```python
from build123d import *

# Parameters (mm, degrees)
F0_R     = 166
F0_R_2   = 140
F1_DEPTH = 49
F2_DEPTH = 49
F3_DEPTH = 22
F4_DEPTH = 43


with BuildPart() as f1:
    # F0 (on Top) → F1 (new body)
    with BuildSketch(Plane.XY):
        Circle(F0_R)
        Circle(F0_R_2, mode=Mode.SUBTRACT)
    extrude(amount=F1_DEPTH)

    # F0 (on Top) → F2 (join)
    with BuildSketch(Plane.XY):
        Circle(F0_R)
        Circle(F0_R_2, mode=Mode.SUBTRACT)
    extrude(amount=-F2_DEPTH)

    # F0 (on Top) → F3 (join)
    with BuildSketch(Plane.XY):
        with BuildLine():
            ThreePointArc((166.7243233605, -38), (169.9277188905, -19.1198941598), (171, 0))
            ThreePointArc((171, 0), (169.9277188905, 19.1198941598), (166.7243233605, 38))
            ThreePointArc((166.7243233605, 38), (120.9152595829, 120.9152595829), (38, 166.7243233605))
            ThreePointArc((38, 166.7243233605), (19.1198941598, 169.9277188905), (0, 171))
            ThreePointArc((0, 171), (-19.1198941598, 169.9277188905), (-38, 166.7243233605))
            ThreePointArc((-38, 166.7243233605), (-120.9152595829, 120.9152595829), (-166.7243233605, 38))
            ThreePointArc((-166.7243233605, 38), (-169.9277188905, 19.1198941598), (-171, 0))
            ThreePointArc((-171, 0), (-169.9277188905, -19.1198941598), (-166.7243233605, -38))
            ThreePointArc((-166.7243233605, -38), (-120.9152595829, -120.9152595829), (-38, -166.7243233605))
            ThreePointArc((-38, -166.7243233605), (-19.1198941598, -169.9277188905), (0, -171))
            ThreePointArc((0, -171), (19.1198941598, -169.9277188905), (38, -166.7243233605))
            ThreePointArc((38, -166.7243233605), (120.9152595829, -120.9152595829), (166.7243233605, -38))
        make_face()
        Circle(F0_R, mode=Mode.SUBTRACT)
        with BuildLine():
            Line((-316, -38), (-166.7243233605, -38))
            ThreePointArc((-166.7243233605, -38), (-169.9277188905, -19.1198941598), (-171, 0))
            Line((-171, 0), (-326, 0))
            ThreePointArc((-326, 0), (-323.4581542767, -19.6468827044), (-316, -38))
        make_face()
        with BuildLine():
            ThreePointArc((-171, 0), (-169.9277188905, 19.1198941598), (-166.7243233605, 38))
            Line((-166.7243233605, 38), (-316, 38))
            ThreePointArc((-316, 38), (-323.4581542767, 19.6468827044), (-326, 0))
            Line((-326, 0), (-171, 0))
        make_face()
        with BuildLine():
            ThreePointArc((-38, 166.7243233605), (-19.1198941598, 169.9277188905), (0, 171))
            Line((0, 171), (0, 326))
            ThreePointArc((0, 326), (-19.6468827044, 323.4581542767), (-38, 316))
            Line((-38, 316), (-38, 166.7243233605))
        make_face()
        with BuildLine():
            ThreePointArc((0, 171), (19.1198941598, 169.9277188905), (38, 166.7243233605))
            Line((38, 166.7243233605), (38, 316))
            ThreePointArc((38, 316), (19.6468827044, 323.4581542767), (0, 326))
            Line((0, 326), (0, 171))
        make_face()
        with BuildLine():
            ThreePointArc((166.7243233605, 38), (169.9277188905, 19.1198941598), (171, 0))
            Line((171, 0), (326, 0))
            ThreePointArc((326, 0), (323.4581542767, 19.6468827044), (316, 38))
            Line((316, 38), (166.7243233605, 38))
        make_face()
        with BuildLine():
            Line((326, 0), (171, 0))
            ThreePointArc((171, 0), (169.9277188905, -19.1198941598), (166.7243233605, -38))
            Line((166.7243233605, -38), (316, -38))
            ThreePointArc((316, -38), (323.4581542767, -19.6468827044), (326, 0))
        make_face()
        with BuildLine():
            Line((38, -316), (38, -166.7243233605))
            ThreePointArc((38, -166.7243233605), (19.1198941598, -169.9277188905), (0, -171))
            Line((0, -171), (0, -326))
            ThreePointArc((0, -326), (19.6468827044, -323.4581542767), (38, -316))
        make_face()
        with BuildLine():
            Line((0, -326), (0, -171))
            ThreePointArc((0, -171), (-19.1198941598, -169.9277188905), (-38, -166.7243233605))
            Line((-38, -166.7243233605), (-38, -316))
            ThreePointArc((-38, -316), (-19.6468827044, -323.4581542767), (0, -326))
        make_face()
    extrude(amount=F3_DEPTH)

    # F0 (on Top) → F4 (join)
    with BuildSketch(Plane.XY):
        with BuildLine():
            ThreePointArc((-171, 0), (-169.9277188905, 19.1198941598), (-166.7243233605, 38))
            Line((-166.7243233605, 38), (-316, 38))
            ThreePointArc((-316, 38), (-323.4581542767, 19.6468827044), (-326, 0))
            Line((-326, 0), (-171, 0))
        make_face()
        with BuildLine():
            Line((-316, -38), (-166.7243233605, -38))
            ThreePointArc((-166.7243233605, -38), (-169.9277188905, -19.1198941598), (-171, 0))
            Line((-171, 0), (-326, 0))
            ThreePointArc((-326, 0), (-323.4581542767, -19.6468827044), (-316, -38))
        make_face()
        with BuildLine():
            ThreePointArc((166.7243233605, -38), (169.9277188905, -19.1198941598), (171, 0))
            ThreePointArc((171, 0), (169.9277188905, 19.1198941598), (166.7243233605, 38))
            ThreePointArc((166.7243233605, 38), (120.9152595829, 120.9152595829), (38, 166.7243233605))
            ThreePointArc((38, 166.7243233605), (19.1198941598, 169.9277188905), (0, 171))
            ThreePointArc((0, 171), (-19.1198941598, 169.9277188905), (-38, 166.7243233605))
            ThreePointArc((-38, 166.7243233605), (-120.9152595829, 120.9152595829), (-166.7243233605, 38))
            ThreePointArc((-166.7243233605, 38), (-169.9277188905, 19.1198941598), (-171, 0))
            ThreePointArc((-171, 0), (-169.9277188905, -19.1198941598), (-166.7243233605, -38))
            ThreePointArc((-166.7243233605, -38), (-120.9152595829, -120.9152595829), (-38, -166.7243233605))
            ThreePointArc((-38, -166.7243233605), (-19.1198941598, -169.9277188905), (0, -171))
            ThreePointArc((0, -171), (19.1198941598, -169.9277188905), (38, -166.7243233605))
            ThreePointArc((38, -166.7243233605), (120.9152595829, -120.9152595829), (166.7243233605, -38))
        make_face()
        Circle(F0_R, mode=Mode.SUBTRACT)
        with BuildLine():
            Line((0, -326), (0, -171))
            ThreePointArc((0, -171), (-19.1198941598, -169.9277188905), (-38, -166.7243233605))
            Line((-38, -166.7243233605), (-38, -316))
            ThreePointArc((-38, -316), (-19.6468827044, -323.4581542767), (0, -326))
        make_face()
        with BuildLine():
            Line((38, -316), (38, -166.7243233605))
            ThreePointArc((38, -166.7243233605), (19.1198941598, -169.9277188905), (0, -171))
            Line((0, -171), (0, -326))
            ThreePointArc((0, -326), (19.6468827044, -323.4581542767), (38, -316))
        make_face()
        with BuildLine():
            Line((326, 0), (171, 0))
            ThreePointArc((171, 0), (169.9277188905, -19.1198941598), (166.7243233605, -38))
            Line((166.7243233605, -38), (316, -38))
            ThreePointArc((316, -38), (323.4581542767, -19.6468827044), (326, 0))
        make_face()
        with BuildLine():
            ThreePointArc((166.7243233605, 38), (169.9277188905, 19.1198941598), (171, 0))
            Line((171, 0), (326, 0))
            ThreePointArc((326, 0), (323.4581542767, 19.6468827044), (316, 38))
            Line((316, 38), (166.7243233605, 38))
        make_face()
        with BuildLine():
            ThreePointArc((0, 171), (19.1198941598, 169.9277188905), (38, 166.7243233605))
            Line((38, 166.7243233605), (38, 316))
            ThreePointArc((38, 316), (19.6468827044, 323.4581542767), (0, 326))
            Line((0, 326), (0, 171))
        make_face()
        with BuildLine():
            ThreePointArc((-38, 166.7243233605), (-19.1198941598, 169.9277188905), (0, 171))
            Line((0, 171), (0, 326))
            ThreePointArc((0, 326), (-19.6468827044, 323.4581542767), (-38, 316))
            Line((-38, 316), (-38, 166.7243233605))
        make_face()
    extrude(amount=-F4_DEPTH)


solid = f1.part
```
Can you work these out from the model? Positions are in its coordinate system, mm. A direction names the side the tool comes from. Give positions to 0.01 mm unless a question says otherwise; leave off trailing zeros. Write each loop counter-clockwise with the first axis right and the second up, starting at its lowest first coordinate (ties: lowest second). Pieces come first, ordered by that corner, then holes. Notation, with made-up numbers: (-9.5, 87) -> (5.5, 87) arc R25 cw to (5.5, 108) -> close; hole circle Ø3 at (60, -18). An arc over 180 degrees is marked (long way). Write item = value, one per line.
(1) Suppose I cut it at D-D on y = -279. Write out the boundary of the cut face in (x, z), then the cut area to 3 significant figures.
Worked out:
outline = (-38, -43) -> (38, -43) -> (38, 22) -> (-38, 22) -> close
area = 4,940 mm^2
(2) Suppose I cut it at A-A on z = 8.5. Write out the boundary of the cut face in (x, y), then the cut area to 3 significant figures.
Worked out:
outline = (-316, -38) -> (-166.72, -38) arc R171 ccw to (-38, -166.72) -> (-38, -316) arc R77.2 ccw to (38, -316) -> (38, -166.72) arc R171 ccw to (166.72, -38) -> (316, -38) arc R77.2 ccw to (316, 38) -> (166.72, 38) arc R171 ccw to (38, 166.72) -> (38, 316) arc R77.2 ccw to (-38, 316) -> (-38, 166.72) arc R171 ccw to (-166.72, 38) -> (-316, 38) arc R77.2 ccw to start; hole circle Ø280 at (0, 0)
area = 76,900 mm^2
(3) I need wall thicknesses on probe 1 along X at (y, z) = (-272, 9); probe 2 along Y at (x, z) = (57.5, 14). Which ranges of each line are inside material? Lowest first, please. Write a range as from..to.
Worked out:
probe_1 = -38..38
probe_2 = -161.04..-127.65, 127.65..161.04
(4) For faces 4 (the face through (-2, -168, 22)), 5 (the face through (-242, -38, -10)), 6 (the face through (-38, 242, -10)), which set-ups out of +Z, -Z, +X, -X, +Y, -Y let a thin tool reach every point of the face, with its end or its side?
Worked out:
face_4 = +Z
face_5 = +Z, -Z, -X, -Y
face_6 = +Z, -Z, -X, +Y
(5) Suppose I cut it at B-B on y = 0. Write out the boundary of the cut face in (x, z), then the cut area to 3 significant figures.
Worked out:
outline = (-326, -43) -> (-166, -43) -> (-166, -49) -> (-140, -49) -> (-140, 49) -> (-166, 49) -> (-166, 22) -> (-326, 22) -> close; (140, -49) -> (166, -49) -> (166, -43) -> (326, -43) -> (326, 22) -> (166, 22) -> (166, 49) -> (140, 49) -> close
area = 25,900 mm^2
(6) Thinking about a two-plate mould opening in Y: for faces 1 (the face through (119.961, -121.862, -10.045)), 2 (the face through (325.998, -0.556, -10.045)), 3 (the face through (-111.1, -85.19, -0.69)), which applies, released by +Y, released by -Y, zero draft, split by the parting line, or undercut?
Worked out:
face_1 = released by -Y
face_2 = split by the parting line
face_3 = undercut
(7) I'm going to push flat-ended pins straight in: P1, Ø6, axis at x = 12, y = -240.5, coming from the -Z side; P2, Ø3, axis at x = -145.5, z = 28.5, coming from the +Y side; P3, Ø12, axis at x = -192.5, z = -34.5, coming from the +Y side. Where does each tip first touch, or does it pass through?
Worked out:
P1 = -43
P2 = 82.58
P3 = 38
